from build123d import *

# Parameters (mm, degrees)
F0_R        = 38.1
F1_DEPTH    = 76.2
F1_TAPER    = 8
F2_W        = 127
F2_H        = 15.875
F3_DEPTH    = 20.32
F4_T        = 2.5
F4_T3_DEPTH = 63.3729932057


# Not quite as in the source:
# - a shell that OpenCascade refuses in one call is made with other operations: the cavity is built on its own and cut out


with BuildPart() as f1:
    # F0 (on Top) → F1 (new body)
    with BuildSketch(Plane.XY):
        Circle(F0_R)
    extrude(amount=F1_DEPTH, taper=F1_TAPER)

    # F2 (on face) → F3 (cut)
    with BuildSketch(Plane.XY.offset(76.2)):
        Rectangle(F2_W, F2_H)
    extrude(amount=-F3_DEPTH, mode=Mode.SUBTRACT)

    # F4: shell of thickness 2.5, made by hand


with BuildPart() as f4_core1:
    # F4_t2: copy of F1
    add(f1.part)

    # the walls: a layer under each face that stays
    f4_faces = [f4_core1.faces().sort_by_distance(p)[0] for p in [
        (-32.7453941978, 0, 38.1),
        (0, 0, 55.88),
        (0, 7.9375, 66.04),
        (0, 17.6641441978, 76.2),
        (0, -7.9375, 66.04),
        (0, -17.6641441978, 76.2),
    ]]
    thicken(f4_faces, amount=-F4_T, mode=Mode.SUBTRACT)

    # F4_s4 → F4_t3 (cut)
    with BuildSketch(Plane.YZ.offset(-31.6864966028)):
        Polygon((7.9125, 55.905), (7.9375, 53.38), (10.4375, 53.38), (10.4375, 55.88), align=None)
        Polygon((-7.9125, 55.905), (-7.9375, 53.38), (-10.4375, 53.38), (-10.4375, 55.88), align=None)
    extrude(amount=F4_T3_DEPTH, mode=Mode.SUBTRACT)


with BuildPart() as f1_1:
    add(f1.part)

    # what is left inside the walls is the cavity
    f4_cavity = [f4_core1.part.solids().sort_by_distance(p)[0] for p in [
        (-32.098055, 0, 24.563187),
    ]]
    add(f4_cavity, mode=Mode.SUBTRACT)


solid = f1_1.part
Model file for the job. Use its own axes, mm. A direction names the side the tool comes from. Give positions to 0.01 mm unless a question says otherwise; leave off trailing zeros. Loops run counter-clockwise (first coordinate to the right, second up) from the corner with the lowest first, then second, coordinate; pieces in that order, holes last. Notation, with made-up numbers: (-11, 60) -> (1, 60) arc R19 ccw to (1, 67) -> close; hole circle Ø6 at (16, 35). An arc over 180 degrees is marked (long way). Use a Markdown table: item, result. Add a question column.
(1) Slice it at A-A on y = 0. List the corners of the cut face in (x, z), and give its area (3 significant figures).
(2) Drop flat-ended pins along their axis: pin 1 Ø2 at (x, z) = (-8, 15.5) entering from +Y; pin 2 Ø6 at (x, y) = (-21.5, 4.5) entering from -Z; pin 3 Ø16.5 at (x, z) = (-12.5, 70) entering from +Y. Give the stop position or say it passes through.
(3) Slice it at D-D on z = 16. List the corners of the cut face in (x, y).
(4) Wall check: line 1 along Y through (x, z) = (-14.5, 65); line 2 along X through (y, z) = (-24, 32); line 3 along X through (y, z) = (-25.5, 5). Give the ranges that are in metal, low to high.
(5) Mould opens along X. For faces 1 (the flat face through (0, -7.938, 66)), 2 (the conical face through (30.18, -12.51, 38.63)), 3 (the flat face through (0, -10.438, 63)) say: +X half, -X half, draft (parallel to the pull), parting line (faces both ways), or undercut.
(6) Slice it at B-B on x = 0. List the corners of the cut face in (y, z), and give its area (3 significant figures).
(7) Tool access for faces 4 (the flat face through (0, 16, 76.2)), 5 (the flat face through (0, 10.438, 63)), 6 (the flat face through (0, 0, 55.88)): list every direction of +Z, -Z, +X, -X, +Y, -Y with a clear straight run to the whole face (end or side of a thin tool).
(8) Slice it at C-C on z = 47.5. List the corners of the cut face in (x, y).
Filled sheet:
| question | item | result |
|---|---|---|
| 1 | outline | (-38.1, 0) -> (-35.58, 0) -> (-28.07, 53.38) -> (28.07, 53.38) -> (35.58, 0) -> (38.1, 0) -> (30.25, 55.88) -> (-30.25, 55.88) -> close |
| 1 | area | 422 mm2 |
| 2 | pin 1 | y = 35.28 |
| 2 | pin 2 | z = 53.38 |
| 2 | pin 3 | y = 28.35 |
| 3 | outline | circle Ø71.7 at (0, 0); hole circle Ø66.65 at (0, 0) |
| 4 | line 1 | -25.07 to -22.11, -10.44 to -7.94, 7.94 to 10.44, 22.11 to 25.07 |
| 4 | line 2 | -23.52 to -19.74, 19.74 to 23.52 |
| 4 | line 3 | -27.36 to -23.79, 23.79 to 27.36 |
| 5 | face 1 | draft |
| 5 | face 2 | parting line |
| 5 | face 3 | undercut |
| 6 | outline | (-38.1, 0) -> (-35.58, 0) -> (-25.22, 73.7) -> (-10.44, 73.7) -> (-10.44, 53.38) -> (10.44, 53.38) -> (10.44, 73.7) -> (25.22, 73.7) -> (35.58, 0) -> (38.1, 0) -> (27.39, 76.2) -> (7.94, 76.2) -> (7.94, 55.88) -> (-7.94, 55.88) -> (-7.94, 76.2) -> (-27.39, 76.2) -> close |
| 6 | area | 612 mm2 |
| 7 | face 4 | +Z, +X, -X, +Y, -Y |
| 7 | face 5 | -Z |
| 7 | face 6 | +Z, +X, -X |
| 8 | outline | circle Ø62.85 at (0, 0); hole circle Ø57.8 at (0, 0) |
